The listing builds one solid part. Answer for the finished solid, in the listing's coordinates (mm). Face numbers are marked on the shaded views. A direction names the side the tool comes from. Coordinates: 2 decimals unless noted, no trailing zeros. Order: outer loops, then holes, each group sorted by start corner. A loop starts at its lowest first (then second) coordinate and runs counter-clockwise, first axis right, second up. Notation, with made-up numbers: (54, 7.5) -> (93, 7.5) arc R15 cw to (93, 14.5) -> close; hole circle Ø1 at (57.5, -13.75). An arc over 180 degrees is marked (long way). Return JSON: item names as keys, results as strings.
```python
from build123d import *

# Parameters (mm, degrees)
SKETCH1_W           = 149
SKETCH1_H           = 75
SKETCH1_R           = 1.65
BOSS_EXTRUDE1_DEPTH = 5
FILLET1_R           = 10
BOSS_EXTRUDE2_DEPTH = 11
BOSS_EXTRUDE3_DEPTH = 2
CHAMFER1_SIZE       = 7.5
BOSS_EXTRUDE4_DEPTH = 5
FILLET2_R           = 3
SKETCH5_W           = 55
SKETCH5_H           = 8
CUT_EXTRUDE1_DEPTH  = 10
FILLET3_R           = 3
FILLET4_R           = 5


with BuildPart() as part:
    # Sketch1 → Boss-Extrude1 (new body)
    with BuildSketch(Plane.XY):
        with Locations((74.5, 37.5)):
            Rectangle(SKETCH1_W, SKETCH1_H)
        with Locations((45, 7.5)):
            Circle(SKETCH1_R, mode=Mode.SUBTRACT)
        with Locations((104, 7.5)):
            Circle(SKETCH1_R, mode=Mode.SUBTRACT)
    extrude(amount=BOSS_EXTRUDE1_DEPTH)

    # Fillet1
    fillet1_edges = [part.edges().sort_by_distance(p)[0] for p in [
        (149, 0, 2.5),
        (0, 0, 2.5),
    ]]
    fillet(fillet1_edges, radius=FILLET1_R)

    # Sketch2 → Boss-Extrude2 (add)
    with BuildSketch(Plane.XY.offset(5)):
        Polygon((0, 75), (2, 75), (2, 73), (2, 32), (147, 32), (147, 55), (149, 55), (149, 30), (0, 30), align=None)
    extrude(amount=BOSS_EXTRUDE2_DEPTH)

    # Sketch3 → Boss-Extrude3 (add)
    with BuildSketch(Plane.XY.offset(16)):
        Polygon((149, 30), (149, 55), (143, 55), (143, 36), (6, 36), (6, 75), (0, 75), (0, 30), align=None)
    extrude(amount=BOSS_EXTRUDE3_DEPTH)

    # Chamfer1
    chamfer1_edges = [part.edges().sort_by_distance(p)[0] for p in [
        (143, 36, 17),
    ]]
    chamfer(chamfer1_edges, length=CHAMFER1_SIZE)

    # Sketch4 → Boss-Extrude4 (add)
    with BuildSketch(Plane.ZY):
        Polygon((18, 30), (5, 18), (5, 30), align=None)
    boss_extrude4 = extrude(amount=-BOSS_EXTRUDE4_DEPTH)

    # Mirror1: Boss-Extrude4 across plane
    add(boss_extrude4.mirror(Plane.ZY.offset(-74.5)))

    # Fillet2
    fillet2_edges = [part.edges().sort_by_distance(p)[0] for p in [
        (146.5, 18, 5),
        (74.5, 30, 5),
        (2.5, 18, 5),
    ]]
    fillet(fillet2_edges, radius=FILLET2_R)

    # Sketch5 → Cut-Extrude1 (cut)
    with BuildSketch(Plane(origin=(0, 32, 0), x_dir=(1, 0, 0), z_dir=(0, 1, 0))):
        with Locations((39.241088115, -10.5)):
            Rectangle(SKETCH5_W, SKETCH5_H)
    extrude(amount=-CUT_EXTRUDE1_DEPTH, mode=Mode.SUBTRACT)

    # Fillet3
    fillet3_edges = [part.edges().sort_by_distance(p)[0] for p in [
        (6, 36, 17),
    ]]
    fillet(fillet3_edges, radius=FILLET3_R)

    # Fillet4
    fillet4_edges = [part.edges().sort_by_distance(p)[0] for p in [
        (149, 75, 2.5),
    ]]
    fillet(fillet4_edges, radius=FILLET4_R)


solid = part.part
```
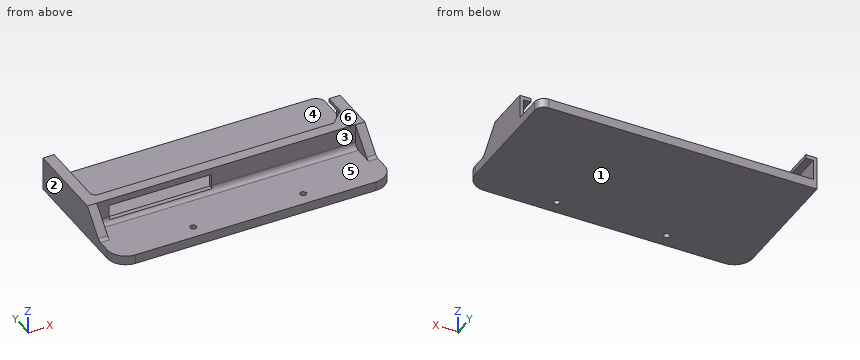
Item 1: The part is cut by section B-B on z = 11. Determine the outline of the cut face in (x, y), plus the area to 3 significant figures.
Answer list:
{"outline": "(0, 23.54) -> (5, 23.54) -> (5, 30) -> (11.74, 30) -> (11.74, 32) -> (2, 32) -> (2, 75) -> (0, 75) -> close; (66.74, 30) -> (144, 30) -> (144, 23.54) -> (149, 23.54) -> (149, 55) -> (147, 55) -> (147, 32) -> (66.74, 32) -> close", "area": "385 mm2"}
Item 2: Determine the mould class of the marked faces 1, 2 and 3 for opening direction X: pulls with the +X half, pulls with the -X half, needs draft (parallel to the pull), parting line crosses it, or undercut.
Answer list:
{"face 1": "needs draft", "face 2": "pulls with the -X half", "face 3": "undercut"}
Item 3: Flat-ended cylindrical pins translate along their axes: pin 1 (1 mm diameter, centred on y = 64.5, z = 17, fed in from +X); pin 2 (4 mm diameter, centred on x = 125, y = 50.5, fed in from +Z); pin 3 (1.5 mm diameter, centred on y = 57.5, z = 9.5, fed in from +X). Find the tip coordinate at first contact, or state that the pin passes through.
Answer list:
{"pin 1": "x = 6", "pin 2": "z = 5", "pin 3": "x = 2"}
Item 4: Which of the six approach directions +Z, -Z, +X, -X, +Y, -Y give full straight-line access (tool end or side, diameter ignored) to the marked faces 4, 5 and 6?
Answer list:
{"face 4": "+Y", "face 5": "+Z, -Y", "face 6": "+Z, +X, -X, +Y, -Y"}
Item 5: Find the intervals of material crossed by probe 1 along Y at (x, z) = (104, 2.6); probe 2 along Z at (x, y) = (67.5, 27); probe 3 along X at (y, z) = (24.5, 9.25), in increasing order.
Answer list:
{"probe 1": "0 to 5.85, 9.15 to 75", "probe 2": "0 to 5", "probe 3": "0 to 5, 144 to 149"}
Item 6: The part is cut by section D-D on y = 7.5. Determine the outline of the cut face in (x, z), plus the area to 3 significant figures.
Answer list:
{"outline": "(0.32, 0) -> (43.35, 0) -> (43.35, 5) -> (0.32, 5) -> close; (46.65, 0) -> (102.35, 0) -> (102.35, 5) -> (46.65, 5) -> close; (105.65, 0) -> (148.68, 0) -> (148.68, 5) -> (105.65, 5) -> close", "area": "709 mm2"}
Item 7: The part is cut by section A-A on x = 104. Determine the outline of the cut face in (y, z), plus the area to 3 significant figures.
Answer list:
{"outline": "(0, 0) -> (5.85, 0) -> (5.85, 5) -> (0, 5) -> close; (9.15, 0) -> (75, 0) -> (75, 5) -> (32, 5) -> (32, 16) -> (36, 16) -> (36, 18) -> (30, 18) -> (30, 8) arc R3 cw to (27, 5) -> (9.15, 5) -> close", "area": "394 mm2"}
Item 8: The part is cut by section C-C on x = 45. Determine the outline of the cut face in (y, z), plus the area to 3 significant figures.
Answer list:
{"outline": "(0, 0) -> (5.85, 0) -> (5.85, 5) -> (0, 5) -> close; (9.15, 0) -> (75, 0) -> (75, 5) -> (32, 5) -> (32, 6.5) -> (29.6, 6.5) arc R3 cw to (27, 5) -> (9.15, 5) -> close; (30, 14.5) -> (32, 14.5) -> (32, 16) -> (36, 16) -> (36, 18) -> (30, 18) -> close", "area": "378 mm2"}
